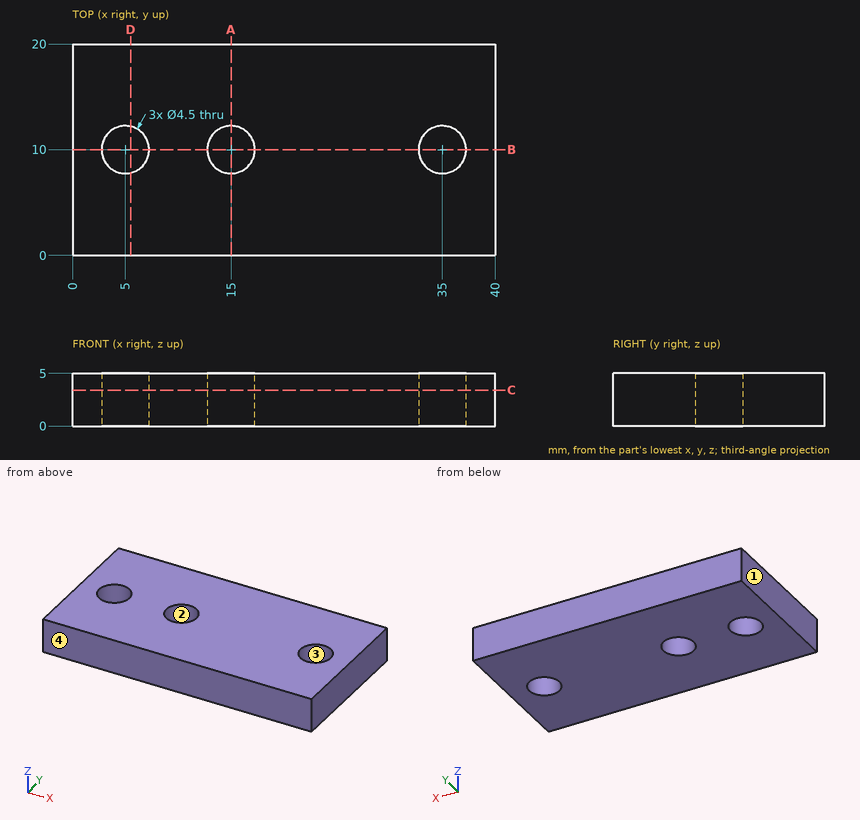
Could you check a few things on this drawing? It's one solid part, dimensions in mm from its lowest x, y, z. Give positions to 0.01 mm unless a question says otherwise; leave off trailing zeros. Write each loop counter-clockwise with the first axis right and the second up, starting at its lowest first coordinate (ties: lowest second). Pieces come first, ordered by that corner, then holes. Notation, with made-up numbers: (-24.5, 66) -> (28.5, 66) arc R11 ccw to (28.5, 84) -> close; hole circle Ø6 at (25.5, -14). An arc over 180 degrees is marked (long way). Write item = value, one per line.
(1) I need wall thicknesses on probe 1 along Y at (x, z) = (35, 3.8); probe 2 along X at (y, z) = (8.75, 0.7); probe 3 along X at (y, z) = (9, 0.75). Which ranges of each line are inside material? Lowest first, please. Write a range as from..to.
Worked out:
probe_1 = 0..7.75, 12.25..20
probe_2 = 0..3.13, 6.87..13.13, 16.87..33.13, 36.87..40
probe_3 = 0..2.98, 7.02..12.98, 17.02..32.98, 37.02..40
(2) Suppose I cut it at C-C on z = 3.4. Write out the boundary of the cut face in (x, y).
Worked out:
outline = (0, 0) -> (40, 0) -> (40, 20) -> (0, 20) -> close; hole circle Ø4.5 at (5, 10); hole circle Ø4.5 at (15, 10); hole circle Ø4.5 at (35, 10)
(3) Suppose I cut it at D-D on x = 5.5. Write out the boundary of the cut face in (y, z).
Worked out:
outline = (0, 0) -> (7.81, 0) -> (7.81, 5) -> (0, 5) -> close; (12.19, 0) -> (20, 0) -> (20, 5) -> (12.19, 5) -> close
(4) Suppose I cut it at B-B on y = 10. Write out the boundary of the cut face in (x, z), then the cut area to 4 significant figures.
Worked out:
outline = (0, 0) -> (2.75, 0) -> (2.75, 5) -> (0, 5) -> close; (7.25, 0) -> (12.75, 0) -> (12.75, 5) -> (7.25, 5) -> close; (17.25, 0) -> (32.75, 0) -> (32.75, 5) -> (17.25, 5) -> close; (37.25, 0) -> (40, 0) -> (40, 5) -> (37.25, 5) -> close
area = 132.5 mm^2
(5) I'm going to push a flat-ended pin straight in: P1, Ø3.5, axis at x = 5, y = 10, coming from the +Z side. Where does the tip first touch, or does it pass through?
Worked out:
P1 = through
(6) Suppose I cut it at A-A on x = 15. Write out the boundary of the cut face in (y, z), then the cut area to 3 significant figures.
Worked out:
outline = (0, 0) -> (7.75, 0) -> (7.75, 5) -> (0, 5) -> close; (12.25, 0) -> (20, 0) -> (20, 5) -> (12.25, 5) -> close
area = 77.5 mm^2
(7) Thinking about a two-plate mould opening in Y: for the marked faces 1, 2, 3 and 4, which applies, released by +Y, released by -Y, zero draft, split by the parting line, or undercut?
Worked out:
face_1 = zero draft
face_2 = undercut
face_3 = undercut
face_4 = released by -Y
